Geometry: final body of the model. Coordinates: model frame, mm. Face numbers are marked on the shaded views. A direction names the side the tool comes from. Coordinates: 2 decimals unless noted, no trailing zeros. Order: outer loops, then holes, each group sorted by start corner. A loop starts at its lowest first (then second) coordinate and runs counter-clockwise, first axis right, second up. Notation, with made-up numbers: M -25,-16.5 L 14,-16.5 A8 ccw 14,-6.5 Z; hole C 5.5,-1 d6. An arc over 180 degrees is marked long. One line per question, with ' | ' between items.
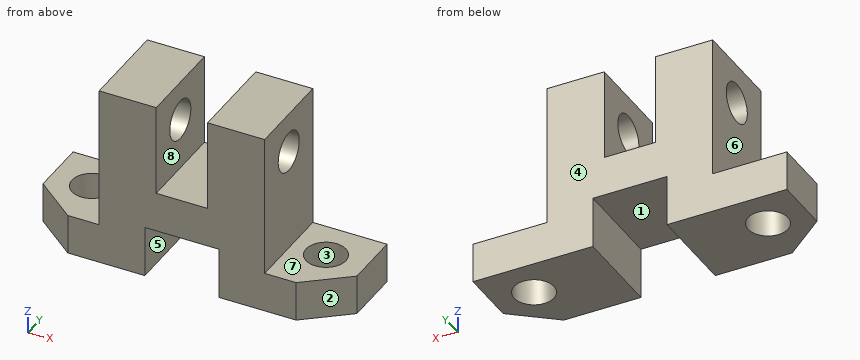
from build123d import *

# Parameters (mm, degrees)
SALIENTE_EXTRUIR1_DEPTH = 32
CROQUIS3_W              = 28.149246734
CROQUIS3_H              = 33.455515618
CORTAR_EXTRUIR1_DEPTH   = 13
CROQUIS4_W              = 32.272758708
CROQUIS4_H              = 29.27783323
CORTAR_EXTRUIR2_DEPTH   = 13
CROQUIS5_W              = 13
CROQUIS5_H              = 9
CORTAR_EXTRUIR3_DEPTH   = 17
CROQUIS6_W              = 9
CROQUIS6_H              = 23
CORTAR_EXTRUIR4_DEPTH   = 17
CROQUIS7_R              = 3.5
CORTAR_EXTRUIR5_DEPTH   = 43
CROQUIS9_R              = 3.5
CORTAR_EXTRUIR6_DEPTH   = 8


with BuildPart() as part:
    # Croquis1 → Saliente-Extruir1 (new body)
    with BuildSketch(Plane.XY):
        Polygon((-20, -11), (-27.5, -5), (-27.5, 5), (27.5, 5), (27.5, -5), (20, -11), align=None)
    extrude(amount=SALIENTE_EXTRUIR1_DEPTH)

    # Croquis3 → Cortar-Extruir1 (cut)
    with BuildSketch(Plane(origin=(27.5, 0, 0), x_dir=(0, 0, -1), z_dir=(1, 0, 0))):
        with Locations((-21.074623367, 0)):
            Rectangle(CROQUIS3_W, CROQUIS3_H)
    extrude(amount=-CORTAR_EXTRUIR1_DEPTH, mode=Mode.SUBTRACT)

    # Croquis4 → Cortar-Extruir2 (cut)
    with BuildSketch(Plane.ZY.offset(27.5)):
        with Locations((23.136379354, -3.846869201)):
            Rectangle(CROQUIS4_W, CROQUIS4_H)
    extrude(amount=-CORTAR_EXTRUIR2_DEPTH, mode=Mode.SUBTRACT)

    # Croquis5 → Cortar-Extruir3 (cut, through all)
    with BuildSketch(Plane.XZ.offset(11)):
        with Locations((0, 4.5)):
            Rectangle(CROQUIS5_W, CROQUIS5_H)
    extrude(amount=-CORTAR_EXTRUIR3_DEPTH, mode=Mode.SUBTRACT)

    # Croquis6 → Cortar-Extruir4 (cut, through all)
    with BuildSketch(Plane.XZ.offset(11)):
        with Locations((0, 27.5)):
            Rectangle(CROQUIS6_W, CROQUIS6_H)
    extrude(amount=-CORTAR_EXTRUIR4_DEPTH, mode=Mode.SUBTRACT)

    # Croquis7 → Cortar-Extruir5 (cut, through all)
    with BuildSketch(Plane(origin=(14.5, 0, 0), x_dir=(0, 0, -1), z_dir=(1, 0, 0))):
        with Locations((-25, -3)):
            Circle(CROQUIS7_R)
    extrude(amount=-CORTAR_EXTRUIR5_DEPTH, mode=Mode.SUBTRACT)

    # Croquis9 → Cortar-Extruir6 (cut, through all)
    with BuildSketch(Plane.XY.offset(7)):
        with Locations((20.5, -2)):
            Circle(CROQUIS9_R)
        with Locations((-20.5, -2)):
            Circle(CROQUIS9_R)
    extrude(amount=-CORTAR_EXTRUIR6_DEPTH, mode=Mode.SUBTRACT)


solid = part.part
1. Material intervals for line 1 (Z direction, x = -13, y = -2.75); line 2 (Y direction, x = -8, z = 25); line 3 (X direction, y = 1.25, z = 21), sorted ascending. Write a range as [from, to].
Response values:
line 1: z = [0, 21.51], [28.49, 32] | line 2: y = [-11, -6.5], [0.5, 5] | line 3: x = [-14.5, -4.5], [4.5, 14.5]
2. Access query for the marked faces 5, 6, 7 and 8. Directions: +Z, -Z, +X, -X, +Y, -Y. A direction counts if a zero-diameter tool reaches every point of the face in a straight line with its end or side. Return the directions, or none.
Response values:
face 5: -Z, +Y, -Y | face 6: +Z, -X, +Y, -Y | face 7: +Z, +X, +Y, -Y | face 8: +Z, +Y, -Y
3. Section C-C, the plane y = -9. Output: boundary loops of the cut face in (x, z), and give its area (3 significant figures).
Response values:
outline: M -22.5,0 L -6.5,0 L -6.5,9 L 6.5,9 L 6.5,0 L 22.5,0 L 22.5,7 L 14.5,7 L 14.5,32 L 4.5,32 L 4.5,16 L -4.5,16 L -4.5,32 L -14.5,32 L -14.5,7 L -22.5,7 Z | area: 779 mm^2
4. Section D-D, the plane z = 18. Output: boundary loops of the cut face in (x, y).
Response values:
outline: M -14.5,-11 L -4.5,-11 L -4.5,5 L -14.5,5 Z; M 4.5,-11 L 14.5,-11 L 14.5,5 L 4.5,5 Z
5. Draft query along Y for the marked faces 1, 2, 3 and 4. Return one class per face: pulls with the +Y half, pulls with the -Y half, needs draft (parallel to the pull), parting line crosses it, or undercut.
Response values:
face 1: needs draft | face 2: pulls with the -Y half | face 3: undercut | face 4: pulls with the +Y half
6. Section A-A, the plane z = 5. Output: boundary loops of the cut face in (x, y).
Response values:
outline: M -27.5,-5 L -20,-11 L -6.5,-11 L -6.5,5 L -27.5,5 Z; M 6.5,-11 L 20,-11 L 27.5,-5 L 27.5,5 L 6.5,5 Z; hole C -20.5,-2 d7; hole C 20.5,-2 d7
7. Section B-B, the plane z = 25. Output: boundary loops of the cut face in (x, y), and give its area (3 significant figures).
Response values:
outline: M -14.5,-11 L -4.5,-11 L -4.5,-6.5 L -14.5,-6.5 Z; M -14.5,0.5 L -4.5,0.5 L -4.5,5 L -14.5,5 Z; M 4.5,-11 L 14.5,-11 L 14.5,-6.5 L 4.5,-6.5 Z; M 4.5,0.5 L 14.5,0.5 L 14.5,5 L 4.5,5 Z | area: 180 mm^2
8. Pin query (flat end, axial travel): P1, Ø5, axis at y = -4, z = 25.5, coming from the -X side; P2, Ø6, axis at y = -1, z = 20, coming from the +X side; P3, Ø9, axis at x = -20.5, y = -2, coming from the +Z side. Return the tip coordinate at first contact, or that it passes through.
Response values:
P1: stops at x = -14.5 | P2: stops at x = 14.5 | P3: stops at z = 7
